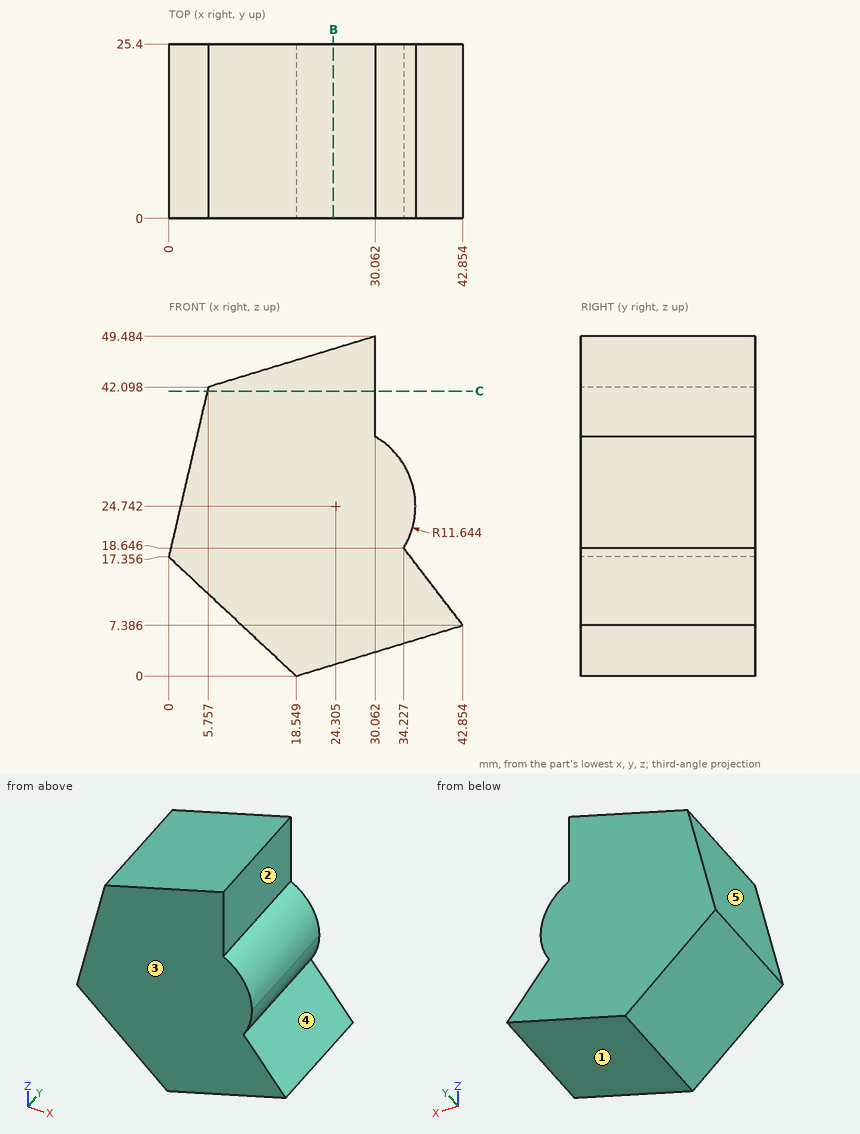
Part print with two shaded views. Sizes in mm from the minimum x, y, z corner. A direction names the side the tool comes from. Round coordinates to 2 decimals unless told otherwise and drop trailing zeros. Write each loop counter-clockwise with the first axis right and the second up, starting at its lowest first coordinate (ties: lowest second). Pieces come first, ordered by that corner, then holes. Notation, with made-up numbers: M 30.25,59.25 L 77.25,59.25 A27 cw 77.25,87.25 Z; hole C 61.5,-27.75 d10. An arc over 180 degrees is marked long. Put each result on its own line as item: value. Start each with the question number.
1) Pin check, flat tips, straight feed: pin 1 Ø2 at (y, z) = (6.5, 15) entering from +X (1 decimal); pin 2 Ø4.5 at (y, z) = (18.5, 42) entering from +X; pin 3 Ø3 at (x, y) = (7.5, 9.5) entering from -Z (1 decimal). Stop position of each tip, or through.
2) Pull direction Z, two halves, no side cores. Call the marked faces 3, 4 and 5: pulls with the +Z half, pulls with the -Z half, needs draft (parallel to the pull), parting line crosses it, or undercut.
3) Saw through at C-C, the plane z = 41.5. Write the cut outline in (x, y).
4) 3-axis set-ups, long thin cutter, end or side, ignore diameter. For the marked faces 1 and 2: which of +Z, -Z, +X, -X, +Y, -Y reach the whole face in a straight line?
5) Saw through at B-B, the plane x = 24. Write the cut outline in (y, z), and give its area (3 significant figures).
6) Drill centre lines: probe 1 along Z at (x, y) = (8, 16.75); probe 2 along X at (y, z) = (4.25, 23); probe 3 along X at (y, z) = (16.5, 33) (1 decimal). Where is each one in solid material? Low to high. Write a range as [from, to].
Resolved:
1. pin 1: x = 37.8
1. pin 2: x = 30.06
1. pin 3: z = 8.9
2. face 3: needs draft
2. face 4: undercut
2. face 5: pulls with the +Z half
3. outline: M 5.62,0 L 30.06,0 L 30.06,25.4 L 5.62,25.4 Z
4. face 1: -Z, +X, +Y, -Y
4. face 2: +Z, +X, +Y, -Y
5. outline: M 0,1.66 L 25.4,1.66 L 25.4,47.64 L 0,47.64 Z
5. area: 1,170 mm²
6. probe 1: [9.87, 42.78]
6. probe 2: [1.31, 35.82]
6. probe 3: [3.6, 32.5]
